```python
from build123d import *

# Parameters (mm, degrees)
F0_W     = 100
F0_H     = 40
F1_DEPTH = 4.5
F2_W     = 100
F2_H     = 40
F2_W_2   = 91
F2_H_2   = 31
F3_DEPTH = 17
F4_R     = 3.277271
F4_R_2   = 2.943444
F4_R_3   = 3.611157
F5_DEPTH = 25


with BuildPart() as f1:
    # F0 (on Top) → F1 (new body)
    with BuildSketch(Plane.XY):
        Rectangle(F0_W, F0_H)
    extrude(amount=F1_DEPTH)

    # F2 (on face) → F3 (join)
    with BuildSketch(Plane.XY.offset(4.5)):
        Rectangle(F2_W, F2_H)
        Rectangle(F2_W_2, F2_H_2, mode=Mode.SUBTRACT)
    extrude(amount=F3_DEPTH)

    # F4 (on face) → F5 (cut)
    with BuildSketch(Plane.XZ.offset(20)):
        with Locations((0, 9.264707)):
            Circle(F4_R)
        with Locations((36.909394, 9.264707)):
            Circle(F4_R_2)
        with Locations((-35.116225, 9.563568)):
            Circle(F4_R_3)
    extrude(amount=-F5_DEPTH, mode=Mode.SUBTRACT)


solid = f1.part
```
For this review, take the finished solid that the model builds, in its own axes (mm). A direction names the side the tool comes from. Coordinates: 2 decimals unless noted, no trailing zeros. Write each loop counter-clockwise with the first axis right and the second up, starting at its lowest first coordinate (ties: lowest second). Pieces come first, ordered by that corner, then holes.
(1) Add section A-A on x = 0. Give the boundary of the cut face in (y, z).
(2) Add section C-C on x = -20. Give the boundary of the cut face in (y, z), then the cut area to 3 significant figures.
(3) For pin 1 Ø5 at (x, y) = (-8.5, 10) entering from +Z; pin 2 Ø5.5 at (x, z) = (36.91, 9.26) entering from -Y, all flat-tipped, find the tip position at first contact; note any pin that passes through.
(4) The part is to be moulded in two halves that separate along Y. For faces 1 (the face through (-1, 20, 11)), 2 (the face through (-1, -20, 13)), 3 (the face through (-1, 15.5, 13)), 4 (the face through (45.5, 0, 13)), say which applies: +Y half, -Y half, draft (parallel to the pull), parting line (faces both ways), or undercut.
(5) Add section D-D on y = -13. Give the boundary of the cut face in (x, z), then the cut area to 3 significant figures.
(6) Tool access review of faces 5 (the face through (-50, 0, 11)), 6 (the face through (33.97, -17.78, 9.39)), 7 (the face through (-1, -15.5, 13)): name each direction out of +Z, -Z, +X, -X, +Y, -Y from which nothing blocks a thin tool from reaching the whole face with its end or side.
(7) Add section B-B on z = 16.5. Give the boundary of the cut face in (x, y), then the cut area to 3 significant figures.
(8) Wall thickness on probe 1 along X at (y, z) = (-6, 7.25); probe 2 along Y at (x, z) = (-39, 13.75); probe 3 along Z at (x, y) = (36, 11): over which ranges is each line inside the solid? List them lowest first.
Answer sheet:
1. outline: (-20, 0) - (20, 0) - (20, 21.5) - (15.5, 21.5) - (15.5, 4.5) - (-15.5, 4.5) - (-15.5, 5.99) - (-20, 5.99) - close; (-20, 12.54) - (-15.5, 12.54) - (-15.5, 21.5) - (-20, 21.5) - close
2. outline: (-20, 0) - (20, 0) - (20, 21.5) - (15.5, 21.5) - (15.5, 4.5) - (-15.5, 4.5) - (-15.5, 21.5) - (-20, 21.5) - close
2. area: 333 mm2
3. pin 1: stops at z = 4.5
3. pin 2: stops at y = 15.5
4. face 1: +Y half
4. face 2: -Y half
4. face 3: undercut
4. face 4: undercut
5. outline: (-50, 0) - (50, 0) - (50, 21.5) - (45.5, 21.5) - (45.5, 4.5) - (-45.5, 4.5) - (-45.5, 21.5) - (-50, 21.5) - close
5. area: 603 mm2
6. face 5: +Z, -Z, -X, +Y, -Y
6. face 6: -Y
6. face 7: +Z
7. outline: (-50, -20) - (50, -20) - (50, 20) - (-50, 20) - close; hole (-45.5, -15.5) - (45.5, -15.5) - (45.5, 15.5) - (-45.5, 15.5) - close
7. area: 1,180 mm2
8. probe 1: x = -50 to -45.5, 45.5 to 50
8. probe 2: y = -20 to -15.5, 15.5 to 20
8. probe 3: z = 0 to 4.5
